Autodesk Inventor part; units mm, degrees
ref_plane "YZ Plane" through (0, 0, 0) normal (1, 0, 0) x (0, 1, 0)
ref_plane "XZ Plane" through (0, 0, 0) normal (0, 1, 0) x (-1, 0, 0)
ref_plane "XY Plane" through (0, 0, 0) normal (0, 0, 1) x (1, 0, 0)
sketch "Sketch1" plane through (0, 0, 0) normal (0, 0, 1) x (1, 0, 0)
  circle A0 centre (0, 0) radius 0.6731
  dimension "d0" = 1.3462
extrude "Extrusion1" add sketch "Sketch1" against normal blind 1.9812
sketch "Sketch2" plane through (0, 0, -1.9812) normal (0, 0, -1) x (-1, 0, 0)
  circle A0 centre (0, 0) radius 1.4224
  dimension "d3" = 2.8448
extrude "Extrusion2" add sketch "Sketch2" along normal blind 4.8006
sketch "Sketch3" plane through (0, 0, -6.7818) normal (0, 0, -1) x (-1, 0, 0)
  circle A0 centre (0, 0) radius 5.2197
  dimension "d6" = 10.4394
extrude "Extrusion3" add sketch "Sketch3" along normal blind 2.9464
sketch "Sketch4" plane through (0, 0, -9.7282) normal (0, 0, -1) x (-1, 0, 0)
  point P0 (0, 0)
sketch "Sketch5" plane through (0, 0, -9.7282) normal (0, 0, -1) x (-1, 0, 0)
  circle A0 centre (0, 0) radius 1.4224
  dimension "d9" = 2.8448
extrude "Extrusion4" add sketch "Sketch5" along normal blind 4.8006
sketch "Sketch6" plane through (0, 0, -14.5288) normal (0, 0, -1) x (-1, 0, 0)
  circle A0 centre (0, 0) radius 0.6731
  dimension "d12" = 1.3462
extrude "Extrusion5" add sketch "Sketch6" along normal blind 1.9812
properties part number "noisemaker"
The model under review builds one solid part; all positions refer to its coordinate system, in mm. A direction names the side the tool comes from. Give positions to 0.01 mm unless a question says otherwise; leave off trailing zeros. Loops run counter-clockwise (first coordinate to the right, second up) from the corner with the lowest first, then second, coordinate; pieces in that order, holes last. Notation, with made-up numbers: (22, 71) -> (71, 71) arc R19 ccw to (71, 100) -> close; hole circle Ø9 at (63.5, -37.5). An arc over 180 degrees is marked (long way). Write each question's results on one line, items separated by ' | '.
1) Take a section at D-D, the plane z = -15. Give the boundary of the cut face in (x, y), plus the area to 3 significant figures.
Conclusion:
outline: circle Ø1.35 at (0, 0) | area: 1.42 mm^2
2) Take a section at C-C, the plane z = -4.5. Give the boundary of the cut face in (x, y), plus the area to 3 significant figures.
Conclusion:
outline: circle Ø2.84 at (0, 0) | area: 6.36 mm^2
3) For line 1 along Z through (x, y) = (1, 3.25); line 2 along X through (y, z) = (4.5, -8.25); line 3 along Y through (x, z) = (-0.5, -12), list the stretches that pass through material, from the lowest coordinate up. Write a range as from..to.
Conclusion:
line 1: z = -9.73..-6.78 | line 2: x = -2.64..2.64 | line 3: y = -1.33..1.33
4) Insertion check: pin 1 Ø6 at (y, z) = (0.5, -13) entering from -X; pin 2 Ø2 at (x, z) = (-1.5, -12) entering from -Y; pin 3 Ø4 at (x, y) = (0, -3.5) entering from -Z. Each pin has a flat end and moves straight along its axis. Give the tip position at first contact, or say it passes through.
Conclusion:
pin 1: stops at x = -1.42 | pin 2: stops at y = -1.33 | pin 3: stops at z = -9.73
5) Tool access review of faces 1 (the face through (-4.82, 2, -8.23)), 2 (the face through (1.2, -1.1, -9.728)), 3 (the face through (0.31, 1.39, -4.35)): name each direction out of +Z, -Z, +X, -X, +Y, -Y from which nothing blocks a thin tool from reaching the whole face with its end or side.
Conclusion:
face 1: +Z, -Z | face 2: -Z | face 3: +Z
6) Take a section at A-A, the plane y = 0. Give the boundary of the cut face in (x, z).
Conclusion:
outline: (-5.22, -9.73) -> (-1.42, -9.73) -> (-1.42, -14.53) -> (-0.67, -14.53) -> (-0.67, -16.51) -> (0.67, -16.51) -> (0.67, -14.53) -> (1.42, -14.53) -> (1.42, -9.73) -> (5.22, -9.73) -> (5.22, -6.78) -> (1.42, -6.78) -> (1.42, -1.98) -> (0.67, -1.98) -> (0.67, 0) -> (-0.67, 0) -> (-0.67, -1.98) -> (-1.42, -1.98) -> (-1.42, -6.78) -> (-5.22, -6.78) -> close
